Input: part model. Units: mm. Frame: model coordinates. A direction names the side the tool comes from. Coordinates: 2 decimals unless noted, no trailing zeros. Write each loop counter-clockwise with the first axis right and the second up, starting at its lowest first coordinate (ties: lowest second). Pieces come first, ordered by that corner, then holes. Notation, with made-up numbers: (10, 62) - (14, 62) arc R29 ccw to (14, 96) - close; hole circle Ø11 at (3.5, 51.5). An arc over 180 degrees is marked (long way). One line per question, with ' | ' between items. Start each with the question number.
1) Draft query along X for faces 5 (the flat face through (13.536, 0.323, 8.395)), 6 (the cylindrical face through (9.277, 15.802, 12.832)), 7 (the cylindrical face through (-7.096, -13.215, 20.055)). Return one class per face: released by +X, released by -X, zero draft, split by the parting line, or undercut.
2) Reachability of faces 1 (the flat face through (-11, 0, 24)), 2 (the flat face through (1.464, 13.677, 8.395)), 3 (the cylindrical face through (21.713, 19.995, 8.395)), 4 (the flat face through (28, 14, 22)) from +Z, -Z, +X, -X, +Y, -Y: full face, straight path, thin tool, end or side. Return the list, or none.
3) Section query B-B on x = 15. Return loops of the section in (y, z), and give its area (3 significant figures).
4) First-contact query: P1, Ø3, axis at y = 14.5, z = 24.5, coming from the +X side; P2, Ø4.5, axis at x = -13, y = -3.5, coming from the +Z side; P3, Ø1.2, axis at x = 28, y = 16.5, coming from the +Z side; P4, Ø1.2, axis at y = 2.5, z = 23.5, coming from the -X side. Flat tips, straight axial feed; report the tip coordinate or a pass-through.
5) Section query C-C on y = 14. Return loops of the section in (x, z), and give its area (3 significant figures).
6) Section query A-A on z = 18.25. Return loops of the section in (x, y), and give its area (3 significant figures).
7) Section query D-D on z = 6.25. Return loops of the section in (x, y).
8) Line query: line 1 (Z direction, x = 27.5, y = 20); line 2 (Z direction, x = 18, y = -1.5); line 3 (X direction, y = 5.5, z = 6). Output: solid intervals per line, ascending.
```python
from build123d import *

# Parameters (mm, degrees)
EXTRUDE_1_DEPTH     = 16
EXTRUDE_2_DEPTH     = 10
CUT_EXTRUDE_1_DEPTH = 4
SKETCH_4_R          = 6
CUT_EXTRUDE_2_DEPTH = 27
CHAMFER_1_SIZE      = 1


with BuildPart() as part:
    # 草图1 → 凸台-拉伸1 (new body)
    with BuildSketch(Plane.XY):
        with BuildLine():
            Line((6.140864253, -6.579497414), (21.140864253, 7.420502586))
            ThreePointArc((21.140864253, 7.420502586), (21.579497414, 20.140864253), (8.859135747, 20.579497414))
            Line((8.859135747, 20.579497414), (-6.140864253, 6.579497414))
            ThreePointArc((-6.140864253, 6.579497414), (-6.579497414, -6.140864253), (6.140864253, -6.579497414))
        make_face()
    extrude(amount=EXTRUDE_1_DEPTH)

    # 草图2 → 凸台-拉伸2 (add)
    with BuildSketch(Plane.XY.offset(16)):
        with BuildLine():
            Line((10.234773755, -10.965829024), (25.234773755, 3.034170976))
            ThreePointArc((25.234773755, 3.034170976), (25.965829024, 24.234773755), (4.765226245, 24.965829024))
            Line((4.765226245, 24.965829024), (-10.234773755, 10.965829024))
            ThreePointArc((-10.234773755, 10.965829024), (-10.965829024, -10.234773755), (10.234773755, -10.965829024))
        make_face()
    extrude(amount=EXTRUDE_2_DEPTH)

    # 草图3 → 切除-拉伸1 (cut)
    with BuildSketch(Plane.XY.offset(26)):
        with BuildLine():
            Line((26, 24.198039027), (26, 3.801960973))
            ThreePointArc((26, 3.801960973), (30, 14), (26, 24.198039027))
        make_face()
        with BuildLine():
            Line((-11, 10.198039027), (-11, -10.198039027))
            ThreePointArc((-11, -10.198039027), (-15, 0), (-11, 10.198039027))
        make_face()
    extrude(amount=-CUT_EXTRUDE_1_DEPTH, mode=Mode.SUBTRACT)

    # 草图4 → 切除-拉伸2 (cut, through all)
    with BuildSketch(Plane(origin=(0, 0, 0), x_dir=(-1, 0, 0), z_dir=(0, 0, -1))):
        Circle(SKETCH_4_R)
        with Locations((-15, 14)):
            Circle(SKETCH_4_R)
    extrude(amount=-CUT_EXTRUDE_2_DEPTH, mode=Mode.SUBTRACT)

    # 倒角1
    chamfer_1_edges = [part.edges().sort_by_distance(p)[0] for p in [
        (-10.965829024, -10.234773755, 16),
        (17.734773755, -3.965829024, 16),
        (25.965829024, 24.234773755, 16),
        (-2.734773755, 17.965829024, 16),
        (-10.624324895, 10.588848876, 26),
        (17.734773755, -3.965829024, 26),
        (25.624324895, 3.411151124, 26),
        (-2.734773755, 17.965829024, 26),
        (-0.542003848, -14.990204529, 26),
        (15.542003848, 28.990204529, 26),
        (1.359135747, 13.579497414, 0),
        (6, 0, 26),
        (6, 0, 0),
        (21, 14, 26),
        (21, 14, 0),
        (21.579497414, 20.140864253, 0),
        (13.640864253, 0.420502586, 0),
        (-6.579497414, -6.140864253, 0),
    ]]
    chamfer(chamfer_1_edges, length=CHAMFER_1_SIZE)


solid = part.part
```
Answer key:
1) face 5: released by +X | face 6: undercut | face 7: split by the parting line
2) face 1: +Z, -X, +Y, -Y | face 2: -Z, -X, +Y | face 3: -Z | face 4: +Z, +X, +Y, -Y
3) outline: (-6.52, 17) - (-5.15, 16) - (1.69, 16) - (1.69, 1) - (3.06, 0) - (7, 0) - (8, 1) - (8, 25) - (7, 26) - (-5.15, 26) - (-6.52, 25) - close; (20, 1) - (21, 0) - (22, 0) - (23, 1) - (23, 16) - (28, 16) - (29, 17) - (29, 25) - (28, 26) - (21, 26) - (20, 25) - close | area: 379 mm²
4) P1: x = 26 | P2: z = 26 | P3: z = 22 | P4: x = -11
5) outline: (-6.98, 17) - (-5.52, 16) - (1.81, 16) - (1.81, 1) - (3.28, 0) - (8, 0) - (9, 1) - (9, 25) - (8, 26) - (-5.52, 26) - (-6.98, 25) - close; (21, 1) - (22, 0) - (23, 0) - (24, 1) - (24, 16) - (29, 16) - (30, 17) - (30, 22) - (26, 22) - (26, 26) - (22, 26) - (21, 25) - close | area: 392 mm²
6) outline: (-10.23, 10.97) arc R15 ccw to (10.23, -10.97) - (25.23, 3.03) arc R15 ccw to (4.77, 24.97) - close; hole circle Ø12 at (0, 0); hole circle Ø12 at (15, 14) | area: 1,100 mm²
7) outline: (-6.14, 6.58) arc R9 ccw to (6.14, -6.58) - (21.14, 7.42) arc R9 ccw to (8.86, 20.58) - close; hole circle Ø12 at (0, 0); hole circle Ø12 at (15, 14)
8) line 1: 16 to 22 | line 2: 16 to 26 | line 3: -7.12 to -2.4, 2.4 to 19.08
